Check sheet for the modelled part. Datum: model origin and axes. Units: mm. Round coordinates to 2 decimals unless told otherwise and drop trailing zeros. Write each loop counter-clockwise with the first axis right and the second up, starting at its lowest first coordinate (ties: lowest second). Pieces come first, ordered by that corner, then holes. Notation, with made-up numbers: (74.5, -16) - (119.5, -16) arc R7 ccw to (119.5, -8) - close; hole circle Ø8 at (41, 5.25). An arc over 180 degrees is marked (long way). Answer as a JSON object with one key per item and string values. Group by question number.
Item 1: Gauge pin test, flat ends, axial feed: P1, Ø2, axis at x = -18.5, z = 1, coming from the +Y side; P2, Ø1, axis at x = 23.5, z = 0.5, coming from the +Y side. Record the tip position at first contact, or that the pin passes through.
Item 2: Thickness scan on line 1 (Z direction, x = -23.5, y = 0.2); line 2 (X direction, y = 1.4, z = -1.25); line 3 (Z direction, x = -26.5, y = 0.6). Record the ranges inside material, lowest first.
Item 3: Sectioned sample at A-A on z = 0. Record the boundary of the cut face in (x, y), plus the area to 3 significant figures.
Item 4: Sectioned sample at D-D on x = 9. Record the boundary of the cut face in (y, z).
Item 5: Sectioned sample at C-C on x = 26.5. Record the boundary of the cut face in (y, z).
```python
from build123d import *


with BuildPart() as part:
    # Sketch4 → Revolve1 (revolve)
    with BuildSketch(Plane(origin=(0, 0, 0), x_dir=(1, 0, 0), z_dir=(0, 1, 0)), mode=Mode.PRIVATE) as revolve1_sk:
        with BuildLine():
            Line((-18, 2), (18, 2))
            ThreePointArc((18, 2), (19.357542477, 1.07262743), (21, 1))
            Line((21, 1), (30, 1))
            Line((30, 1), (30, 0))
            Line((30, 0), (-30, 0))
            Line((-30, 0), (-30, 1))
            Line((-30, 1), (-21, 1))
            ThreePointArc((-21, 1), (-19.357542477, 1.07262743), (-18, 2))
        make_face()
    revolve(revolve1_sk.sketch.rotate(Axis((-30, 0, 0), (1, 0, 0)), 180), axis=Axis((-30, 0, 0), (1, 0, 0)))


solid = part.part
```
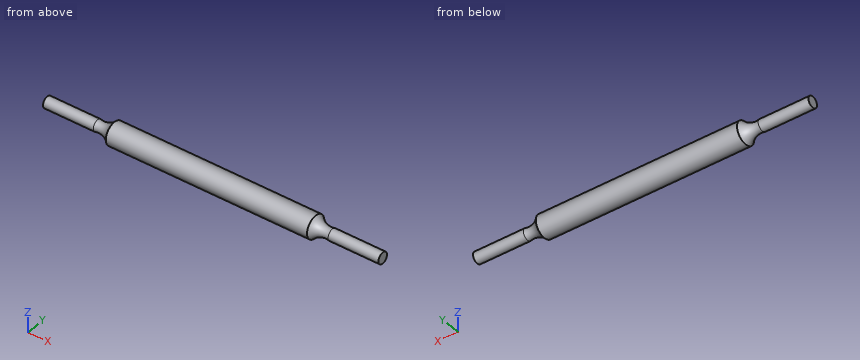
Completed:
{
 "1": {"P1": "y = 2", "P2": "y = 1"},
 "2": {"line 1": "-0.98 to 0.98", "line 2": "-18.11 to 18.11", "line 3": "-0.8 to 0.8"},
 "3": {"outline": "(-30, -1) - (-21, -1) arc R3 cw to (-18, -2) - (18, -2) arc R3 cw to (21, -1) - (30, -1) - (30, 1) - (21, 1) arc R3 cw to (18, 2) - (-18, 2) arc R3 cw to (-21, 1) - (-30, 1) - close", "area": "194 mm²"},
 "4": {"outline": "circle Ø4 at (0, 0)"},
 "5": {"outline": "circle Ø2 at (0, 0)"}
}
